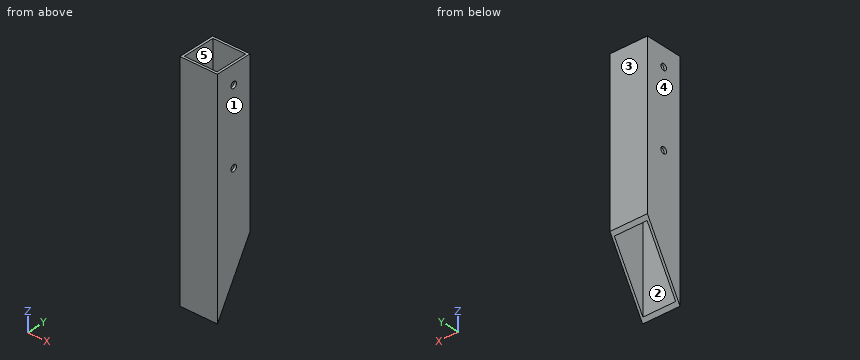
```python
from build123d import *

# Parameters (mm, degrees)
F0_W     = 25.4
F0_H     = 25.4
F0_W_2   = 22.225
F0_H_2   = 22.225
F1_DEPTH = 152.4
F3_DEPTH = 25.4
F4_R     = 2.15265
F5_DEPTH = 25.4


with BuildPart() as f1:
    # F0 (on Top) → F1 (new body)
    with BuildSketch(Plane.XY):
        Rectangle(F0_W, F0_H)
        Rectangle(F0_W_2, F0_H_2, mode=Mode.SUBTRACT)
    extrude(amount=F1_DEPTH)

    # F2 (on face) → F3 (cut, through all)
    with BuildSketch(Plane.YZ.offset(12.7)):
        Polygon((12.7, 43.994091), (-12.7, 0), (12.7, 0), align=None)
    extrude(amount=-F3_DEPTH, mode=Mode.SUBTRACT)

    # F4 (on face) → F5 (cut, through all)
    with BuildSketch(Plane.YZ.offset(12.7)):
        with Locations((0, 139.7)):
            Circle(F4_R)
        with Locations((0, 88.9)):
            Circle(F4_R)
    extrude(amount=-F5_DEPTH, mode=Mode.SUBTRACT)


solid = f1.part
```
Part model, mm, in its own coordinate system. Face numbers are marked on the shaded views. A direction names the side the tool comes from. Round coordinates to 2 decimals unless told otherwise and drop trailing zeros. Write each loop counter-clockwise with the first axis right and the second up, starting at its lowest first coordinate (ties: lowest second). Pieces come first, ordered by that corner, then holes. Notation, with made-up numbers: M -15.75,-19.5 L 16.25,-19.5 A34 cw 16.25,18.5 Z; hole C -9.75,71.25 d2. An arc over 180 degrees is marked long. Answer as CSV lines item,"result". Start each with the question number.
1) Which spindle directions (+Z, -Z, +X, -X, +Y, -Y) get a long thin tool onto all of the face, cutting with end or side? Do the marked faces 4 and 5. Say none if no direction does.
2) Band-saw the part on C-C (y = -7.75). List the corners of the cut face in (x, z), then the cut area to 3 significant figures.
3) Drill centre lines: L1, parallel to X at y = 4.25, z = 89.5; L2, parallel to Y at x = 12.1, z = 139.7. Where is each one in solid material? Low to high.
4) Band-saw the part on D-D (z = 63). List the corners of the cut face in (x, y), then the cut area to 3 significant figures.
5) Band-saw the part on B-B (x = -6.75). List the corners of the cut face in (y, z).
6) Band-saw the part on A-A (z = 139.7). List the corners of the cut face in (x, y).
7) Mould opens along Y. For the marked faces 1, 2 and 3 say: +Y half, -Y half, draft (parallel to the pull), parting line (faces both ways), or undercut.
Worked out:
1,face 4,"+Z, -Z, -X, +Y, -Y"
1,face 5,"+Z, -Z"
2,outline,"M -12.7,8.57 L -11.11,8.57 L -11.11,152.4 L -12.7,152.4 Z; M 11.11,8.57 L 12.7,8.57 L 12.7,152.4 L 11.11,152.4 Z"
2,area,"457 mm²"
3,L1,"-12.7 to -11.11, 11.11 to 12.7"
3,L2,"-12.7 to -2.15, 2.15 to 12.7"
4,outline,"M -12.7,-12.7 L 12.7,-12.7 L 12.7,12.7 L -12.7,12.7 Z; hole M -11.11,-11.11 L 11.11,-11.11 L 11.11,11.11 L -11.11,11.11 Z"
4,area,"151 mm²"
5,outline,"M -12.7,0 L -11.11,2.75 L -11.11,152.4 L -12.7,152.4 Z; M 11.11,41.24 L 12.7,43.99 L 12.7,152.4 L 11.11,152.4 Z"
6,outline,"M -12.7,-12.7 L 12.7,-12.7 L 12.7,-2.15 L 11.11,-2.15 L 11.11,-11.11 L -11.11,-11.11 L -11.11,-2.15 L -12.7,-2.15 Z; M -12.7,2.15 L -11.11,2.15 L -11.11,11.11 L 11.11,11.11 L 11.11,2.15 L 12.7,2.15 L 12.7,12.7 L -12.7,12.7 Z"
7,face 1,"draft"
7,face 2,"undercut"
7,face 3,"+Y half"
